Check sheet for the modelled part. Datum: model origin and axes. Units: mm. A direction names the side the tool comes from. Coordinates: 2 decimals unless noted, no trailing zeros. Loops run counter-clockwise (first coordinate to the right, second up) from the corner with the lowest first, then second, coordinate; pieces in that order, holes last. Notation, with made-up numbers: (28, 76.5) - (37, 76.5) arc R26 cw to (37, 113.5) - close; hole circle Ø8 at (65.5, -29). An arc over 180 degrees is marked (long way). Use a Markdown table: item, result. Add a question column.
1) Go/stop test with flat-tipped pins: P1, Ø5, axis at x = -15.5, y = 15.5, coming from the +Z side; P2, Ø8, axis at y = 4.5, z = -34, coming from the +X side; P3, Ø1.5, axis at x = -16.5, z = -20, coming from the -Y side. Record where each tip stops, or that it passes through.
2) Tool access check on faces 1 (the flat face through (-19, 17, -39.25)), 2 (the cylindrical face through (-17.623, -17.732, -24.214)), 3 (the flat face through (-21.109, 0, -24)), 4 (the flat face through (0, -21.109, -24)), 5 (the cylindrical face through (-15.57, -14, -2.96)). Record the directions out of +Z, -Z, +X, -X, +Y, -Y that give a thin tool (end or side, any length) a straight path to the whole face; none if there is none.
3) Thickness scan on line 1 (Y direction, x = -15.5, z = -1.15); line 2 (X direction, y = 15, z = -2). Record the ranges inside material, lowest first.
4) Sectioned sample at D-D, the plane y = 12. Enter the section's corners in (x, z).
5) Sectioned sample at B-B, the plane y = 0. Enter the section's corners in (x, z), then the cut area to 3 significant figures.
6) Draft check along Y on faces 6 (the flat face through (21.109, 0, -24)), 7 (the cylindrical face through (14.49, -14.39, -2.96)), 8 (the cylindrical face through (-16.345, 16.421, -5.26)), 9 (the cylindrical face through (18.701, -18.776, -43.686)). Enter one of: pulls with the +Y half, pulls with the -Y half, needs draft (parallel to the pull), parting line crosses it, or undercut.
7) Sectioned sample at C-C, the plane x = 0. Enter the section's corners in (y, z).
8) Sectioned sample at A-A, the plane z = -20.5. Enter the section's corners in (x, y).
from build123d import *

# Parameters (mm, degrees)
SKETCH1_R                      = 2.5
BOSS_EXTRUDE1_DEPTH            = 24
SKETCH2_R                      = 11
BOSS_EXTRUDE2_DEPTH            = 2
SKETCH3_W                      = 42.418
SKETCH3_H                      = 42.418
BOSS_EXTRUDE3_DEPTH            = 48
CUT_EXTRUDE1_DEPTH             = 73
M3X0_5_TAPPED_HOLE1_AT_2_COUNT = 2
M3X0_5_TAPPED_HOLE1_AT_2_PITCH = 31
M3X0_5_TAPPED_HOLE1_AT_3_COUNT = 2
M3X0_5_TAPPED_HOLE1_AT_3_PITCH = 43.840620434
M3X0_5_TAPPED_HOLE1_AT_4_COUNT = 2
M3X0_5_TAPPED_HOLE1_AT_4_PITCH = 31
CUT_EXTRUDE2_DEPTH             = 15
CUT_EXTRUDE3_DEPTH             = 15.25
CUT_EXTRUDE3_DEPTH_BACK        = 15.25


with BuildPart() as part:
    # Sketch1 → Boss-Extrude1 (new body)
    with BuildSketch(Plane.XY):
        Circle(SKETCH1_R)
    extrude(amount=BOSS_EXTRUDE1_DEPTH)

    # Sketch2 → Boss-Extrude2 (add)
    with BuildSketch(Plane(origin=(0, 0, 0), x_dir=(-1, 0, 0), z_dir=(0, 0, -1))):
        Circle(SKETCH2_R)
    extrude(amount=-BOSS_EXTRUDE2_DEPTH)

    # Sketch3 → Boss-Extrude3 (add)
    with BuildSketch(Plane(origin=(0, 0, 0), x_dir=(-1, 0, 0), z_dir=(0, 0, -1))):
        Rectangle(SKETCH3_W, SKETCH3_H)
    extrude(amount=BOSS_EXTRUDE3_DEPTH)

    # Sketch4 → Cut-Extrude1 (cut, through all)
    with BuildSketch(Plane(origin=(0, 0, -48), x_dir=(-1, 0, 0), z_dir=(0, 0, -1))):
        with BuildLine():
            Line((-21.209, -15.887992919), (-21.209, -21.209))
            Line((-21.209, -21.209), (-15.887992919, -21.209))
            ThreePointArc((-15.887992919, -21.209), (-18.738329701, -18.738329701), (-21.209, -15.887992919))
        make_face()
        with BuildLine():
            Line((15.887992919, -21.209), (21.209, -21.209))
            Line((21.209, -21.209), (21.209, -15.887992919))
            ThreePointArc((21.209, -15.887992919), (18.738329701, -18.738329701), (15.887992919, -21.209))
        make_face()
        with BuildLine():
            Line((21.209, 15.887992919), (21.209, 21.209))
            Line((21.209, 21.209), (15.887992919, 21.209))
            ThreePointArc((15.887992919, 21.209), (18.738329701, 18.738329701), (21.209, 15.887992919))
        make_face()
        with BuildLine():
            Line((-15.887992919, 21.209), (-21.209, 21.209))
            Line((-21.209, 21.209), (-21.209, 15.887992919))
            ThreePointArc((-21.209, 15.887992919), (-18.738329701, 18.738329701), (-15.887992919, 21.209))
        make_face()
    extrude(amount=-CUT_EXTRUDE1_DEPTH, mode=Mode.SUBTRACT)

    # Sketch5 → M3x0.5 Tapped Hole1 (revolve, cut)
    with BuildSketch(Plane(origin=(-15.5, 15.5, 0), x_dir=(0, -1, 0), z_dir=(1, 0, 0))):
        Polygon((0, 0), (0, 5.251075774), (1.25, 4.5), (1.25, 6), (1.5, 6), (1.5, 0), align=None)
    m3x0_5_tapped_hole1 = revolve(axis=Axis((-15.5, 15.5, 6.35), (0, 0, -1)), mode=Mode.SUBTRACT)

    # M3x0.5 Tapped Hole1 at 2: M3x0.5 Tapped Hole1 ×2
    with Locations(*[(0, -i * M3X0_5_TAPPED_HOLE1_AT_2_PITCH, 0) for i in range(1, M3X0_5_TAPPED_HOLE1_AT_2_COUNT)]):
        add(m3x0_5_tapped_hole1, mode=Mode.SUBTRACT)

    # M3x0.5 Tapped Hole1 at 3: M3x0.5 Tapped Hole1 ×2
    with Locations(*[Vector(0.707106781, -0.707106781, 0) * (i * M3X0_5_TAPPED_HOLE1_AT_3_PITCH) for i in range(1, M3X0_5_TAPPED_HOLE1_AT_3_COUNT)]):
        add(m3x0_5_tapped_hole1, mode=Mode.SUBTRACT)

    # M3x0.5 Tapped Hole1 at 4: M3x0.5 Tapped Hole1 ×2
    with Locations(*[(i * M3X0_5_TAPPED_HOLE1_AT_4_PITCH, 0, 0) for i in range(1, M3X0_5_TAPPED_HOLE1_AT_4_COUNT)]):
        add(m3x0_5_tapped_hole1, mode=Mode.SUBTRACT)

    # Sketch7 → Cut-Extrude2 (cut)
    with BuildSketch(Plane.XY.offset(24)):
        with BuildLine():
            Line((-1.5, 2), (1.5, 2))
            ThreePointArc((1.5, 2), (0, 2.5), (-1.5, 2))
        make_face()
    extrude(amount=-CUT_EXTRUDE2_DEPTH, mode=Mode.SUBTRACT)

    # Sketch8 → Cut-Extrude3 (cut, two sides)
    with BuildSketch(Plane.XY.offset(-24)) as cut_extrude3_sk:
        with BuildLine():
            Line((15.887992919, 21.209), (-15.887992919, 21.209))
            ThreePointArc((-15.887992919, 21.209), (-18.738329701, 18.738329701), (-21.209, 15.887992919))
            Line((-21.209, 15.887992919), (-21.209, -15.887992919))
            ThreePointArc((-21.209, -15.887992919), (-18.738329701, -18.738329701), (-15.887992919, -21.209))
            Line((-15.887992919, -21.209), (15.887992919, -21.209))
            ThreePointArc((15.887992919, -21.209), (18.738329701, -18.738329701), (21.209, -15.887992919))
            Line((21.209, -15.887992919), (21.209, 15.887992919))
            ThreePointArc((21.209, 15.887992919), (18.738329701, 18.738329701), (15.887992919, 21.209))
        make_face()
        with BuildLine():
            Line((-13.394406258, 21.109), (13.394406258, 21.109))
            ThreePointArc((13.394406258, 21.109), (17.67766953, 17.67766953), (21.109, 13.394406258))
            Line((21.109, 13.394406258), (21.109, -13.394406258))
            ThreePointArc((21.109, -13.394406258), (17.67766953, -17.67766953), (13.394406258, -21.109))
            Line((13.394406258, -21.109), (-13.394406258, -21.109))
            ThreePointArc((-13.394406258, -21.109), (-17.67766953, -17.67766953), (-21.109, -13.394406258))
            Line((-21.109, -13.394406258), (-21.109, 13.394406258))
            ThreePointArc((-21.109, 13.394406258), (-17.67766953, 17.67766953), (-13.394406258, 21.109))
        make_face(mode=Mode.SUBTRACT)
    extrude(amount=CUT_EXTRUDE3_DEPTH, mode=Mode.SUBTRACT)
    extrude(cut_extrude3_sk.sketch, amount=-CUT_EXTRUDE3_DEPTH_BACK, mode=Mode.SUBTRACT)


solid = part.part
Solved:
| question | item | result |
|---|---|---|
| 1 | P1 | stops at z = 0 |
| 1 | P2 | stops at x = 21.11 |
| 1 | P3 | stops at y = -19.41 |
| 2 | face 1 | none |
| 2 | face 2 | -X, -Y |
| 2 | face 3 | -X, +Y, -Y |
| 2 | face 4 | +X, -X, -Y |
| 2 | face 5 | +Z |
| 3 | line 1 | y = -21.21 to -17, -14 to 14, 17 to 21.21 |
| 3 | line 2 | x = -21.21 to -16.91, -14.09 to 14.09, 16.91 to 21.21 |
| 4 | outline | (-21.21, -48) - (21.21, -48) - (21.21, -39.25) - (21.11, -39.25) - (21.11, -8.75) - (21.21, -8.75) - (21.21, 0) - (-21.21, 0) - (-21.21, -8.75) - (-21.11, -8.75) - (-21.11, -39.25) - (-21.21, -39.25) - close |
| 5 | outline | (-21.21, -48) - (21.21, -48) - (21.21, -39.25) - (21.11, -39.25) - (21.11, -8.75) - (21.21, -8.75) - (21.21, 0) - (11, 0) - (11, 2) - (2.5, 2) - (2.5, 24) - (-2.5, 24) - (-2.5, 2) - (-11, 2) - (-11, 0) - (-21.21, 0) - (-21.21, -8.75) - (-21.11, -8.75) - (-21.11, -39.25) - (-21.21, -39.25) - close |
| 5 | area | 2,180 mm2 |
| 6 | face 6 | needs draft |
| 6 | face 7 | undercut |
| 6 | face 8 | undercut |
| 6 | face 9 | pulls with the -Y half |
| 7 | outline | (-21.21, -48) - (21.21, -48) - (21.21, -39.25) - (21.11, -39.25) - (21.11, -8.75) - (21.21, -8.75) - (21.21, 0) - (11, 0) - (11, 2) - (2.5, 2) - (2.5, 9) - (2, 9) - (2, 24) - (-2.5, 24) - (-2.5, 2) - (-11, 2) - (-11, 0) - (-21.21, 0) - (-21.21, -8.75) - (-21.11, -8.75) - (-21.11, -39.25) - (-21.21, -39.25) - close |
| 8 | outline | (-21.11, -13.39) arc R25 ccw to (-13.39, -21.11) - (13.39, -21.11) arc R25 ccw to (21.11, -13.39) - (21.11, 13.39) arc R25 ccw to (13.39, 21.11) - (-13.39, 21.11) arc R25 ccw to (-21.11, 13.39) - close |
